Autodesk Inventor part; units mm, degrees
ref_plane "Work Plane1" through (60.2053, -12.7096, 92.2812) normal (0, 1, 0) x (-1, 0, 0)
ref_plane "YZ Plane" through (0, 0, 0) normal (1, 0, 0) x (0, 1, 0)
ref_plane "XZ Plane" through (0, 0, 0) normal (0, 1, 0) x (-1, 0, 0)
ref_plane "Work Plane1" through (60.2053, -12.7096, 92.2812) normal (0, 1, 0) x (-1, 0, 0)
sketch "Sketch1" plane through (60.2053, -12.7096, 92.2812) normal (0, 1, 0) x (-1, 0, 0)
  arc A0 (-40.6666, -82.6341) -> (-12.2349, -84.0587) centre (-25.049, -55.3704) ccw construction
  arc A1 (12.2349, -84.0587) -> (-12.2349, -84.0587) centre (0, -111.4504) ccw construction
  arc A2 (12.2349, -84.0587) -> (40.6666, -82.6341) centre (25.049, -55.3704) ccw construction
  arc A3 (40.6666, -82.6341) -> (81.8144, -11.6423) centre (0, -11.6423) ccw construction
  line L0 (81.8144, -11.6423) -> (81.8144, 75.1302) construction
  arc A4 (81.8144, 75.1302) -> (81.2286, 76.5444) centre (79.8144, 75.1302) ccw construction
  line L1 (81.2286, 76.5444) -> (71.5684, 86.2046) construction
  arc A5 (71.5684, 86.2046) -> (70.1542, 86.7904) centre (70.1542, 84.7904) ccw construction
  line L2 (70.1542, 86.7904) -> (-70.1542, 86.7904) construction
  arc A6 (-70.1542, 86.7904) -> (-71.5684, 86.2046) centre (-70.1542, 84.7904) ccw construction
  line L3 (-71.5684, 86.2046) -> (-81.2286, 76.5444) construction
  arc A7 (-81.2286, 76.5444) -> (-81.8144, 75.1302) centre (-79.8144, 75.1302) ccw construction
  line L4 (-81.8144, 75.1302) -> (-81.8144, -11.6423) construction
  arc A8 (-81.8144, -11.6423) -> (-40.6666, -82.6341) centre (0, -11.6423) ccw construction
  arc A9 (10, -81.3229) -> (-10, -81.3229) centre (0, -11.6423) ccw construction
  arc A10 (-39.9607, -81.4019) -> (-10, -81.3229) centre (-25.049, -55.3704) ccw construction
  arc A11 (-80.3944, -11.6423) -> (-39.9607, -81.4019) centre (0, -11.6423) ccw construction
  line L5 (-80.3944, 75.3704) -> (-80.3944, -11.6423) construction
  line L6 (-70.3944, 85.3704) -> (-80.3944, 75.3704) construction
  line L7 (70.3944, 85.3704) -> (-70.3944, 85.3704) construction
  line L8 (80.3944, 75.3704) -> (70.3944, 85.3704) construction
  line L9 (80.3944, -11.6423) -> (80.3944, 75.3704) construction
  arc A12 (39.9607, -81.4019) -> (80.3944, -11.6423) centre (0, -11.6423) ccw construction
  arc A13 (10, -81.3229) -> (39.9607, -81.4019) centre (25.049, -55.3704) ccw construction
  circle A14 centre (0, -11.6423) radius 68.3944 construction
  arc A15 (-87.3944, -11.6423) -> (87.3944, -11.6423) centre (0, -11.6423) ccw construction
  line L10 (87.3944, 88.3704) -> (87.3944, -11.6423) construction
  arc A16 (87.3944, 88.3704) -> (83.3944, 92.3704) centre (83.3944, 88.3704) ccw construction
  line L11 (-83.3944, 92.3704) -> (83.3944, 92.3704) construction
  arc A17 (-83.3944, 92.3704) -> (-87.3944, 88.3704) centre (-83.3944, 88.3704) ccw construction
  line L12 (-87.3944, -11.6423) -> (-87.3944, 88.3704) construction
  circle A18 centre (0, -95.5368) radius 1.85 construction
  circle A19 centre (-83.3944, 88.3704) radius 1.85 construction
  circle A20 centre (83.3944, 88.3704) radius 1.85 construction
  arc A21 (-85.9744, -11.6423) -> (-42.7343, -86.2438) centre (0, -11.6423) ccw construction
  line L13 (-85.9744, -11.6423) -> (-85.9744, 75.1302) construction
  arc A22 (-84.1702, 79.486) -> (-85.9744, 75.1302) centre (-79.8144, 75.1302) ccw construction
  line L14 (-84.1702, 79.486) -> (-74.51, 89.1462) construction
  arc A23 (-70.1542, 90.9504) -> (-74.51, 89.1462) centre (-70.1542, 84.7904) ccw construction
  line L15 (-70.1542, 90.9504) -> (70.1542, 90.9504) construction
  arc A24 (74.51, 89.1462) -> (70.1542, 90.9504) centre (70.1542, 84.7904) ccw construction
  line L16 (74.51, 89.1462) -> (84.1702, 79.486) construction
  arc A25 (85.9744, 75.1302) -> (84.1702, 79.486) centre (79.8144, 75.1302) ccw construction
  line L17 (85.9744, 75.1302) -> (85.9744, -11.6423) construction
  arc A26 (42.7343, -86.2438) -> (85.9744, -11.6423) centre (0, -11.6423) ccw construction
  arc A27 (10.5384, -87.857) -> (42.7343, -86.2438) centre (25.049, -55.3704) ccw construction
  arc A28 (10.5384, -87.857) -> (-10.5384, -87.857) centre (0, -111.4504) ccw construction
  arc A29 (-42.7343, -86.2438) -> (-10.5384, -87.857) centre (-25.049, -55.3704) ccw construction
  line L18 (-83.8944, -11.6423) -> (-83.8944, 75.1302)
  arc A30 (-82.6994, 78.0152) -> (-83.8944, 75.1302) centre (-79.8144, 75.1302) ccw
  line L19 (-82.6994, 78.0152) -> (-73.0392, 87.6754)
  arc A31 (-70.1542, 88.8704) -> (-73.0392, 87.6754) centre (-70.1542, 84.7904) ccw
  line L20 (-70.1542, 88.8704) -> (70.1542, 88.8704)
  arc A32 (73.0392, 87.6754) -> (70.1542, 88.8704) centre (70.1542, 84.7904) ccw
  line L21 (73.0392, 87.6754) -> (82.6994, 78.0152)
  arc A33 (83.8944, 75.1302) -> (82.6994, 78.0152) centre (79.8144, 75.1302) ccw
  line L22 (83.8944, 75.1302) -> (83.8944, -11.6423)
  arc A34 (41.7004, -84.439) -> (83.8944, -11.6423) centre (0, -11.6423) ccw
  arc A35 (11.3866, -85.9579) -> (41.7004, -84.439) centre (25.049, -55.3704) ccw
  arc A36 (11.3866, -85.9579) -> (-11.3866, -85.9579) centre (0, -111.4504) ccw
  arc A37 (-41.7004, -84.439) -> (-11.3866, -85.9579) centre (-25.049, -55.3704) ccw
  arc A38 (-83.8944, -11.6423) -> (-41.7004, -84.439) centre (0, -11.6423) ccw
  point P0 (60.2053, -92.2812)
  dimension "d0" = 2.08
sketch "Sketch2" plane through (0, 0, 0) normal (1, 0, 0) x (0, 1, 0)
  circle A0 centre (-12.7096, 181.1516) radius 2.5
  point P0 (0, 0)
  dimension "d1" = 5
sweep "Sweep1" add profiles "Sketch2" path "Sketch1"
properties part number "middle_gasket" material "Rubber, Black"
Check sheet for the modelled part. Datum: model origin and axes. Units: mm. Give positions to 0.01 mm unless a question says otherwise; leave off trailing zeros. Order: outer loops, then holes, each group sorted by start corner. A loop starts at its lowest first (then second) coordinate and runs counter-clockwise, first axis right, second up. Notation, with made-up numbers: (34, -28.75) - (65, -28.75) arc R23 cw to (65, -8.75) - close; hole circle Ø11 at (39.25, -5). An arc over 180 degrees is marked (long way). Answer as CSV lines item,"result".
1. Go/stop test with flat-tipped pins: P1, Ø2, axis at x = 76, y = -11.5, coming from the +Z side; P2, Ø3, axis at y = -14.5, z = 56.5, coming from the +X side. Record where each tip stops, or that it passes through.
Result sheet:
P1,"z = 183.64"
P2,"x = 143.35"
2. Scan lines: probe 1 along X at (y, z) = (-13.05, 131.5); probe 2 along Z at (x, y) = (2.5, -13.4); probe 3 along Z at (x, y) = (78, -14.55). Record each from-to range of solid material in increasing order. Write a range as from..to.
Result sheet:
probe 1,"-26.17..-21.21, 141.62..146.58"
probe 2,"16.47..23.1, 178.75..183.55"
probe 3,"2.47..5.94, 179.46..182.84"
3. Section check A-A (z = 115). Record the boundary of the cut face in (x, y), then the cut area to 3 significant figures.
Result sheet:
outline,"circle Ø5 at (-23.69, -12.71); circle Ø5 at (144.1, -12.71)"
area,"39.3 mm²"
